Here's how the part is built. I have some questions about the finished solid (model axes, mm). A direction names the side the tool comes from. Give positions to 0.01 mm unless a question says otherwise; leave off trailing zeros. Loops run counter-clockwise (first coordinate to the right, second up) from the corner with the lowest first, then second, coordinate; pieces in that order, holes last. Notation, with made-up numbers: (67.5, 24) - (76.5, 24) arc R19 cw to (76.5, 51) - close; hole circle Ø8 at (76.5, 73.5). An arc over 180 degrees is marked (long way). Use a Markdown table: item, result.
from build123d import *

# Parameters (mm, degrees)
SKETCH1_R           = 9.35
SKETCH1_R_2         = 2.5
BOSS_EXTRUDE1_DEPTH = 25
SKETCH2_R           = 4
CUT_EXTRUDE1_DEPTH  = 12.5
SKETCH3_R           = 1.5
CUT_EXTRUDE2_DEPTH  = 8
CIRPATTERN1_COUNT   = 2
CIRPATTERN1_ANGLE   = 90


with BuildPart() as part:
    # Sketch1 → Boss-Extrude1 (new body)
    with BuildSketch(Plane(origin=(0, 0, 0), x_dir=(1, 0, 0), z_dir=(0, 1, 0))):
        with Locations(Location((0, 0, 0), (0, 0, 270))):
            Circle(SKETCH1_R)
        with Locations(Location((0, 0, 0), (0, 0, 270))):
            Circle(SKETCH1_R_2, mode=Mode.SUBTRACT)
    extrude(amount=BOSS_EXTRUDE1_DEPTH)

    # Sketch2 → Cut-Extrude1 (cut)
    with BuildSketch(Plane(origin=(0, 25, 0), x_dir=(1, 0, 0), z_dir=(0, 1, 0))):
        with Locations(Location((0, 0, 0), (0, 0, 270))):
            Circle(SKETCH2_R)
    extrude(amount=-CUT_EXTRUDE1_DEPTH, mode=Mode.SUBTRACT)

    # Sketch3 → Cut-Extrude2 (cut)
    with BuildSketch(Plane.ZY.offset(9.35)):
        with Locations((0, 21)):
            Circle(SKETCH3_R)
        with Locations((0, 4)):
            Circle(SKETCH3_R)
    cut_extrude2 = extrude(amount=-CUT_EXTRUDE2_DEPTH, mode=Mode.SUBTRACT)

    # CirPattern1: Cut-Extrude2 ×2 about axis
    cirpattern1_axis = Axis((0, 12.5, 0), (0, -1, 0))
    for i in range(1, CIRPATTERN1_COUNT):
        add(cut_extrude2.rotate(cirpattern1_axis, i * CIRPATTERN1_ANGLE / (CIRPATTERN1_COUNT - 1)), mode=Mode.SUBTRACT)


solid = part.part
(1) Suppose I cut it at A-A on z = 0. Write out the boundary of the cut face in (x, y).
A:
| item | result |
|---|---|
| outline | (-9.35, 0) - (-2.5, 0) - (-2.5, 2.5) - (-9.35, 2.5) - close; (-9.35, 5.5) - (-2.5, 5.5) - (-2.5, 12.5) - (-4, 12.5) - (-4, 19.5) - (-9.35, 19.5) - close; (-9.35, 22.5) - (-4, 22.5) - (-4, 25) - (-9.35, 25) - close; (2.5, 0) - (9.35, 0) - (9.35, 25) - (4, 25) - (4, 12.5) - (2.5, 12.5) - close |
(2) Suppose I cut it at D-D on x = -4.75. Write out the boundary of the cut face in (y, z), plus the area to 3 significant figures.
A:
| item | result |
|---|---|
| outline | (0, -8.05) - (25, -8.05) - (25, 8.05) - (0, 8.05) - close; hole circle Ø3 at (4, 0); hole circle Ø3 at (21, 0) |
| area | 389 mm2 |
(3) We'd pull the mould along X, two halves only. Please class faces 1 (the face through (2.808, 12.325, 8.918)), 2 (the face through (2, 12.5, 2)), 3 (the face through (-2, 0, 2)): pulls with the +X half, pulls with the -X half, needs draft (parallel to the pull), parting line crosses it, or undercut.
A:
| item | result |
|---|---|
| face 1 | parting line crosses it |
| face 2 | undercut |
| face 3 | needs draft |
(4) Suppose I cut it at C-C on z = -3. Write out the boundary of the cut face in (x, y).
A:
| item | result |
|---|---|
| outline | (-8.86, 0) - (8.86, 0) - (8.86, 25) - (2.65, 25) - (2.65, 12.5) - (-2.65, 12.5) - (-2.65, 25) - (-8.86, 25) - close; hole circle Ø3 at (0, 4) |
(5) Suppose I cut it at B-B on y = 21. Write out the boundary of the cut face in (x, z).
A:
| item | result |
|---|---|
| outline | (-9.23, -1.5) arc R9.35 ccw to (-1.5, -9.23) - (-1.5, -3.71) arc R4 cw to (-3.71, -1.5) - close; (-9.23, 1.5) - (-3.71, 1.5) arc R4 cw (long way) to (1.5, -3.71) - (1.5, -9.23) arc R9.35 ccw (long way) to start |
(6) Will these pins go through, and if not, where does the flat tip stop? pin 1 (5 mm diameter, centred on x = -6, y = 3.5, fed in from +Z); pin 2 (10 mm diameter, centred on x = 7.5, y = 19, fed in from -Z); pin 3 (1 mm diameter, centred on x = -2, y = 12.5, fed in from +Z).
A:
| item | result |
|---|---|
| pin 1 | z = 8.67 |
| pin 2 | z = -9.01 |
| pin 3 | z = 9.23 |
(7) On a 3-axis mill with a long thin cutter (end or side, diameter ignored), from which of +Z, -Z, +X, -X, +Y, -Y can I reach the whole of each face in a straight line? I mean faces 4 (the face through (1.201, 18.838, 3.815)), 5 (the face through (-6.568, 22.487, -0.195)), 6 (the face through (2.11, 6.16, 1.34)), 7 (the face through (-1.43, 4.45, -5.73)), 8 (the face through (-4, 25, 2)). Say none if no direction works.
A:
| item | result |
|---|---|
| face 4 | +Y |
| face 5 | -X |
| face 6 | +Y, -Y |
| face 7 | -Z |
| face 8 | +Z, -Z, +X, -X, +Y |
(8) If I drill on line 1 (Y direction, x = -7.85, z = 0); line 2 (Z direction, x = 0, y = 7); line 3 (Y direction, x = -0.75, z = -7), over which ranges is the centre line in solid material (lowest first)?
A:
| item | result |
|---|---|
| line 1 | 0 to 2.5, 5.5 to 19.5, 22.5 to 25 |
| line 2 | -9.35 to -2.5, 2.5 to 9.35 |
| line 3 | 0 to 2.7, 5.3 to 19.7, 22.3 to 25 |
